```python
from build123d import *

# Parameters (mm, degrees)
SKETCH1_W                = 28
SKETCH1_H                = 15.8
BASE_DEPTH               = 10.4
SKETCH2_W                = 0.8
SKETCH2_H                = 7.7
END_PRONGS_DEPTH         = 12
SKETCH3_W                = 12
SKETCH3_H                = 7.7
SIDE_PRONG_EXTRUDE_DEPTH = 4
SKETCH4_W                = 11.2
SKETCH4_H                = 3.2
SIDE_PRONG_CUT_DEPTH     = 44.949317401
SKETCH6_R                = 1.6
SKETCH6_R_2              = 2.365004953
HOLES_DEPTH              = 45.247033799
SKETCH5_W                = 16.481894615
SKETCH5_H                = 5
BOSS_EXTRUDE4_DEPTH      = 9.2
SKETCH7_W                = 9.2
SKETCH7_H                = 5
BOSS_EXTRUDE5_DEPTH      = 10


with BuildPart() as part:
    # Sketch1 → Base (new body)
    with BuildSketch(Plane(origin=(0, 0, 0), x_dir=(1, 0, 0), z_dir=(0, 1, 0))):
        with Locations((14, 7.9)):
            Rectangle(SKETCH1_W, SKETCH1_H)
    extrude(amount=BASE_DEPTH)

    # Sketch2 → End Prongs (add)
    with BuildSketch(Plane(origin=(28, 0, 0), x_dir=(0, 0, -1), z_dir=(1, 0, 0))):
        with Locations((5.2, 5.2)):
            Rectangle(SKETCH2_W, SKETCH2_H)
        with Locations((10.6, 5.2)):
            Rectangle(SKETCH2_W, SKETCH2_H)
    extrude(amount=END_PRONGS_DEPTH)

    # Sketch3 → Side Prong Extrude (add)
    with BuildSketch(Plane.XY):
        with Locations((21, 5.2)):
            Rectangle(SKETCH3_W, SKETCH3_H)
    extrude(amount=SIDE_PRONG_EXTRUDE_DEPTH)

    # Sketch4 → Side Prong Cut (cut, through all)
    with BuildSketch(Plane(origin=(0, 9.05, 0), x_dir=(1, 0, 0), z_dir=(0, 1, 0))):
        with Locations((21.4, -1.6)):
            Rectangle(SKETCH4_W, SKETCH4_H)
    extrude(amount=-SIDE_PRONG_CUT_DEPTH, mode=Mode.SUBTRACT)

    # Sketch6 → Holes (cut, through all)
    with BuildSketch(Plane(origin=(0, 10.4, 0), x_dir=(1, 0, 0), z_dir=(0, 1, 0))):
        with Locations(Location((25, 13.1, 0), (0, 0, 270))):
            Circle(SKETCH6_R)
        with Locations(Location((3, 2.8, 0), (0, 0, 270))):
            Circle(SKETCH6_R_2)
    extrude(amount=-HOLES_DEPTH, mode=Mode.SUBTRACT)

    # Sketch5 → Boss-Extrude4 (add)
    with BuildSketch(Plane(origin=(0, 0, -15.8), x_dir=(-1, 0, 0), z_dir=(0, 0, -1))):
        with Locations((-8.240947308, 5.589136769)):
            Rectangle(SKETCH5_W, SKETCH5_H)
    extrude(amount=BOSS_EXTRUDE4_DEPTH)

    # Sketch7 → Boss-Extrude5 (add)
    with BuildSketch(Plane.ZY):
        with Locations((-20.4, 5.589136769)):
            Rectangle(SKETCH7_W, SKETCH7_H)
    extrude(amount=BOSS_EXTRUDE5_DEPTH)


solid = part.part
```
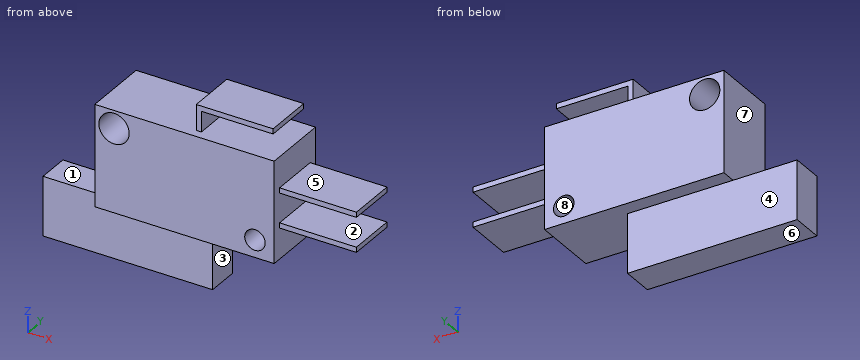
CAD build for the part. Positions are in the model's coordinates, mm. Face numbers are marked on the shaded views. A direction names the side the tool comes from. Give positions to 0.01 mm unless a question says otherwise; leave off trailing zeros. Loops run counter-clockwise (first coordinate to the right, second up) from the corner with the lowest first, then second, coordinate; pieces in that order, holes last. Notation, with made-up numbers: (-22.75, 38) -> (12.25, 38) arc R17 ccw to (12.25, 42) -> close; hole circle Ø8 at (51.5, 87.25). An arc over 180 degrees is marked (long way). Use a Markdown table: item, result.
1. Slice it at D-D (x = 11). List the corners of the cut face in (y, z), plus the area to 3 significant figures.
Check result:
| item | result |
|---|---|
| outline | (0, -15.8) -> (3.09, -15.8) -> (3.09, -25) -> (8.09, -25) -> (8.09, -15.8) -> (10.4, -15.8) -> (10.4, 0) -> (0, 0) -> close |
| area | 210 mm^2 |
2. Which spindle directions (+Z, -Z, +X, -X, +Y, -Y) get a long thin tool onto all of the face, cutting with end or side? Do the marked faces 1, 2, 3, 4 and 5. Say none if no direction does.
Check result:
| item | result |
|---|---|
| face 1 | +Z, -X, +Y, -Y |
| face 2 | +X, +Y, -Y |
| face 3 | -Z, +X, +Y, -Y |
| face 4 | -Z, +X, -X, +Y |
| face 5 | +Z, +X, +Y, -Y |
3. Slice it at A-A (x = 30.5). List the corners of the cut face in (y, z), plus the area to 3 significant figures.
Check result:
| item | result |
|---|---|
| outline | (1.35, -11) -> (9.05, -11) -> (9.05, -10.2) -> (1.35, -10.2) -> close; (1.35, -5.6) -> (9.05, -5.6) -> (9.05, -4.8) -> (1.35, -4.8) -> close |
| area | 12.3 mm^2 |
4. Slice it at B-B (z = -2.8). List the corners of the cut face in (x, y) (3 decimals).
Check result:
| item | result |
|---|---|
| outline | (0, 0) -> (0.635, 0) -> (0.635, 10.4) -> (0, 10.4) -> close; (5.365, 0) -> (28, 0) -> (28, 10.4) -> (5.365, 10.4) -> close |
5. Flat gauge pins, fed straight in: pin 1 (2 mm diameter, centred on y = 6.5, z = -18, fed in from +X); pin 2 (1.5 mm diameter, centred on x = -2, z = 0.5, fed in from +Y); pin 3 (2 mm diameter, centred on x = 23, z = 2.5, fed in from -Y); pin 4 (2.5 mm diameter, centred on x = 37, y = 6, fed in from +Z). Where does each tip first touch, or does it go through?
Check result:
| item | result |
|---|---|
| pin 1 | stops at x = 16.48 |
| pin 2 | passes through |
| pin 3 | stops at y = 1.35 |
| pin 4 | stops at z = -4.8 |
6. Mould opens along X. For the marked faces 6, 7 and 8 say: pulls with the +X half, pulls with the -X half, needs draft (parallel to the pull), parting line crosses it, or undercut.
Check result:
| item | result |
|---|---|
| face 6 | needs draft |
| face 7 | pulls with the -X half |
| face 8 | undercut |
7. Slice it at C-C (y = 6.75). List the corners of the cut face in (x, z) (3 decimals).
Check result:
| item | result |
|---|---|
| outline | (-10, -25) -> (16.482, -25) -> (16.482, -15.8) -> (28, -15.8) -> (28, -11) -> (40, -11) -> (40, -10.2) -> (28, -10.2) -> (28, -5.6) -> (40, -5.6) -> (40, -4.8) -> (28, -4.8) -> (28, 0) -> (15.8, 0) -> (15.8, 3.2) -> (27, 3.2) -> (27, 4) -> (15, 4) -> (15, 0) -> (0, 0) -> (0, -15.8) -> (-10, -15.8) -> close; hole circle Ø4.73 at (3, -2.8); hole circle Ø3.2 at (25, -13.1) |
8. Wall check: L1, parallel to Z at x = 33, y = 8.5; L2, parallel to Z at x = 25.5, y = 1.5; L3, parallel to X at y = 7, z = -13.1. Give the ranges that are in metal, low to high. Write a range as [from, to].
Check result:
| item | result |
|---|---|
| L1 | z = [-11, -10.2], [-5.6, -4.8] |
| L2 | z = [-15.8, -14.62], [-11.58, 0], [3.2, 4] |
| L3 | x = [0, 23.4], [26.6, 28] |
